Here's the drawing with two shaded views (mm, measured from the low corner). I have some questions. Coordinates: 2 decimals unless noted, no trailing zeros. Write each loop counter-clockwise with the first axis right and the second up, starting at its lowest first coordinate (ties: lowest second). Pieces come first, ordered by that corner, then holes.
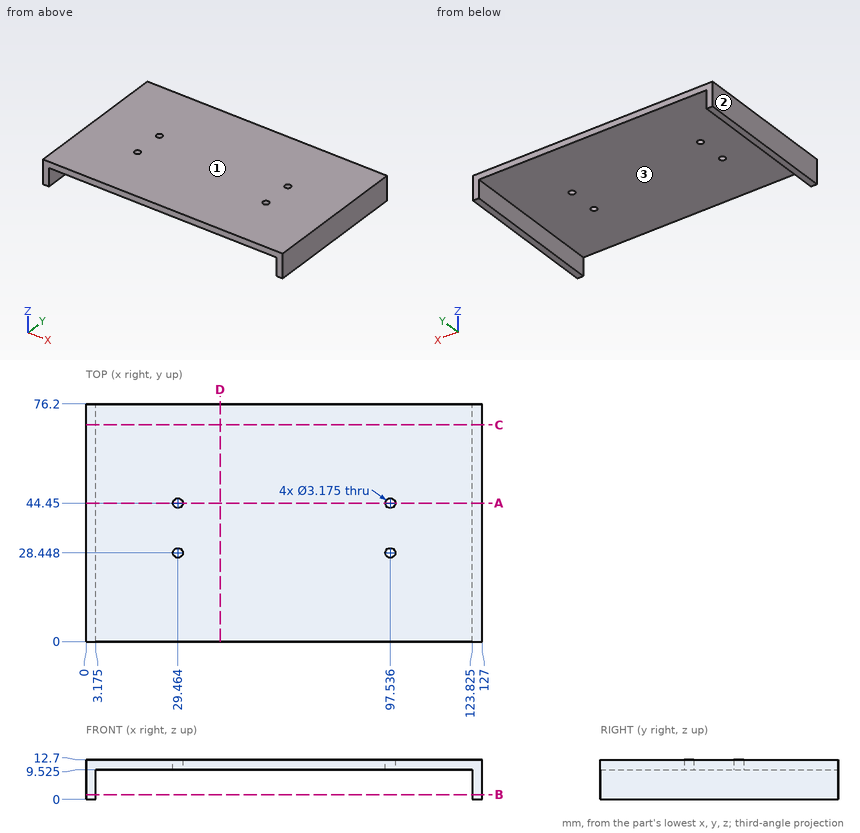
Item 1: If we mould it in two halves opening along Z, with no side actions, what happens to the marked faces 1, 2 and 3? For each: released by +Z, released by -Z, zero draft, split by the parting line, or undercut.
Item 2: Will these pins go through, and if not, where does the flat tip stop? pin 1 Ø5 at (x, y) = (29.464, 44.45) entering from -Z (3 decimals); pin 2 Ø3.5 at (x, y) = (97.536, 44.45) entering from +Z.
Item 3: I want a section at D-D, the plane x = 43. List the corners of the cut face in (y, z) for me (3 decimals), then the cut area to 3 significant figures.
Item 4: I want a section at C-C, the plane y = 69.5. List the corners of the cut face in (x, z) for me (3 decimals), then the cut area to 3 significant figures.
Item 5: I want a section at A-A, the plane y = 44.45. List the corners of the cut face in (x, z) for me (1 decimal).
Item 6: I want a section at B-B, the plane z = 1.5. List the corners of the cut face in (x, y) for me (3 decimals), then the cut area to 3 significant figures.
Item 7: If I drill on line 1 along X through (y, z) = (48, 2.5) (3 decimals); line 2 along X through (y, z) = (45, 10); line 3 along Z through (x, y) = (39, 57) (3 decimals), over which ranges is the centre line in solid material (lowest first)?
Taken from the geometry:
1. face 1: released by +Z
1. face 2: zero draft
1. face 3: released by -Z
2. pin 1: stops at z = 9.525
2. pin 2: stops at z = 12.7
3. outline: (0, 9.525) - (76.2, 9.525) - (76.2, 12.7) - (0, 12.7) - close
3. area: 242 mm2
4. outline: (0, 0) - (3.175, 0) - (3.175, 9.525) - (123.825, 9.525) - (123.825, 0) - (127, 0) - (127, 12.7) - (0, 12.7) - close
4. area: 464 mm2
5. outline: (0, 0) - (3.2, 0) - (3.2, 9.5) - (27.9, 9.5) - (27.9, 12.7) - (0, 12.7) - close; (31.1, 9.5) - (95.9, 9.5) - (95.9, 12.7) - (31.1, 12.7) - close; (99.1, 9.5) - (123.8, 9.5) - (123.8, 0) - (127, 0) - (127, 12.7) - (99.1, 12.7) - close
6. outline: (0, 0) - (3.175, 0) - (3.175, 76.2) - (0, 76.2) - close; (123.825, 0) - (127, 0) - (127, 76.2) - (123.825, 76.2) - close
6. area: 484 mm2
7. line 1: x = 0 to 3.175, 123.825 to 127
7. line 2: x = 0 to 27.97, 30.95 to 96.05, 99.03 to 127
7. line 3: z = 9.525 to 12.7
